The drawing under review shows one solid part. Ordinate dimensions are in mm from its lowest x, y, z. A direction names the side the tool comes from. Round coordinates to 2 decimals unless told otherwise and drop trailing zeros. Loops run counter-clockwise (first coordinate to the right, second up) from the corner with the lowest first, then second, coordinate; pieces in that order, holes last. Notation, with made-up numbers: M 38.25,-18.75 L 91.25,-18.75 A16 ccw 91.25,11.25 Z; hole C 13.25,21.5 d3. An arc over 180 degrees is marked long. Use a Markdown table: item, result.
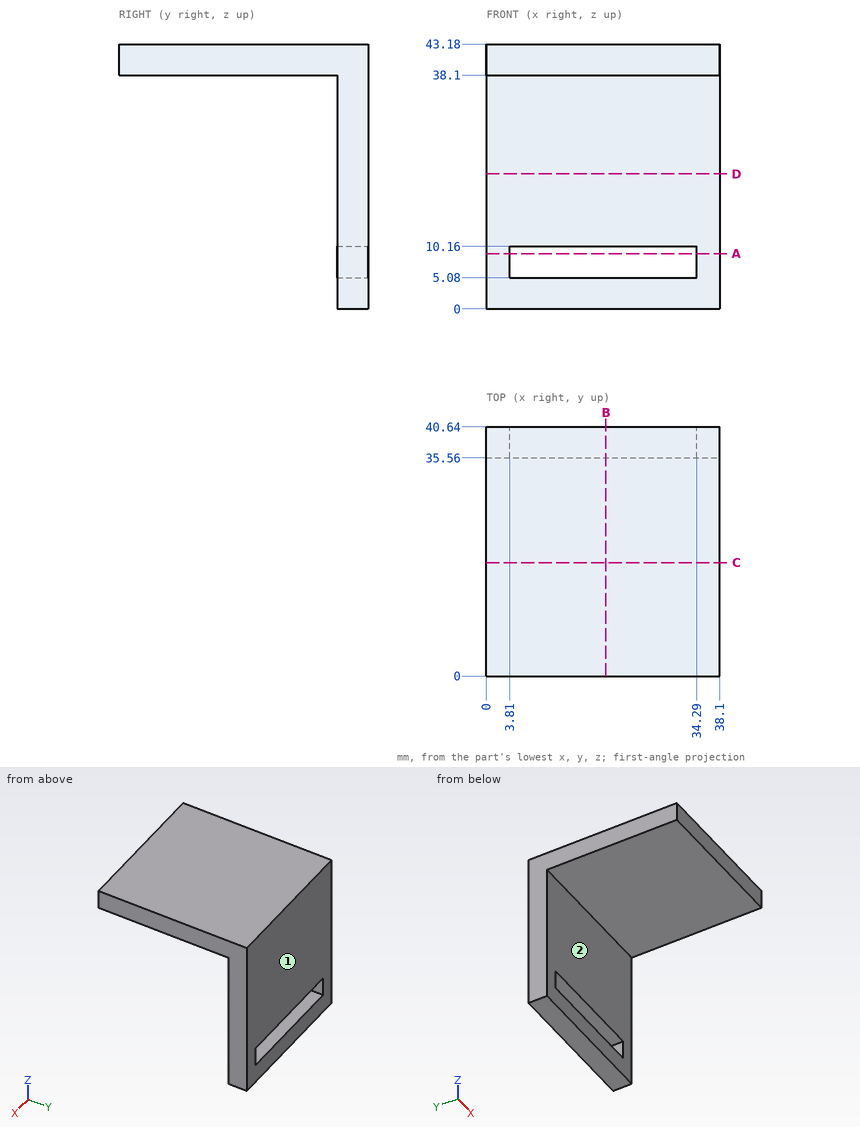
1. Insertion check: pin 1 (11.5 mm diameter, centred on x = 10, z = 10, fed in from -Y); pin 2 (8 mm diameter, centred on x = 18.5, y = 17, fed in from -Z). Each pin has a flat end and moves straight along its axis. Give the tip position at first contact, or say it passes through.
Check values:
| item | result |
|---|---|
| pin 1 | stops at y = 35.56 |
| pin 2 | stops at z = 38.1 |
2. Take a section at B-B on x = 19.5. Give the boundary of the cut face in (y, z), and give its area (3 significant figures).
Check values:
| item | result |
|---|---|
| outline | M 0,38.1 L 35.56,38.1 L 35.56,10.16 L 40.64,10.16 L 40.64,43.18 L 0,43.18 Z; M 35.56,0 L 40.64,0 L 40.64,5.08 L 35.56,5.08 Z |
| area | 374 mm² |
3. Take a section at C-C on y = 18.5. Give the boundary of the cut face in (x, z), and give its area (3 significant figures).
Check values:
| item | result |
|---|---|
| outline | M 0,38.1 L 38.1,38.1 L 38.1,43.18 L 0,43.18 Z |
| area | 194 mm² |
4. Take a section at A-A on z = 9. Give the boundary of the cut face in (x, y).
Check values:
| item | result |
|---|---|
| outline | M 0,35.56 L 3.81,35.56 L 3.81,40.64 L 0,40.64 Z; M 34.29,35.56 L 38.1,35.56 L 38.1,40.64 L 34.29,40.64 Z |
5. Wall thickness on line 1 along Z through (x, y) = (13, 36); line 2 along Y through (x, z) = (13, 25.5); line 3 along Z through (x, y) = (20, 32): over which ranges is each line inside the solid? List them lowest first. Write a range as from..to.
Check values:
| item | result |
|---|---|
| line 1 | z = 0..5.08, 10.16..43.18 |
| line 2 | y = 35.56..40.64 |
| line 3 | z = 38.1..43.18 |
6. Machinability: for the marked faces 1 and 2, which of the approach directions +Z, -Z, +X, -X, +Y, -Y give a long, thin tool a straight path to every point of the face, cutting with its end or side? Answer none if there is none.
Check values:
| item | result |
|---|---|
| face 1 | +Z, -Z, +X, -X, +Y |
| face 2 | -Z, +X, -X, -Y |
7. Take a section at D-D on z = 22. Give the boundary of the cut face in (x, y).
Check values:
| item | result |
|---|---|
| outline | M 0,35.56 L 38.1,35.56 L 38.1,40.64 L 0,40.64 Z |
